Geometry: final body of the model. Coordinates: model frame, mm. A direction names the side the tool comes from. Round coordinates to 2 decimals unless told otherwise and drop trailing zeros. Loops run counter-clockwise (first coordinate to the right, second up) from the corner with the lowest first, then second, coordinate; pieces in that order, holes last. Notation, with made-up numbers: M 83.5,-32 L 126.5,-32 A31 cw 126.5,-7 Z; hole C 79,-4.75 d3. An arc over 180 degrees is marked long. Answer as a JSON object with one key per item and string values.
Autodesk Inventor part; units mm, degrees
ref_plane "YZ Plane" through (0, 0, 0) normal (1, 0, 0) x (0, 1, 0)
ref_plane "XZ Plane" through (0, 0, 0) normal (0, 1, 0) x (-1, 0, 0)
ref_plane "XY Plane" through (0, 0, 0) normal (0, 0, 1) x (1, 0, 0)
sketch "Sketch1" plane through (0, 0, 0) normal (0, 1, 0) x (-1, 0, 0)
  circle A0 centre (0, 0) radius 22.2885
  dimension "d0" = 44.577
extrude "Extrusion1" add sketch "Sketch1" along normal blind 12.7
chamfer "Chamfer1" distance 0.7384 angle 45 1 edges at (22.2885, 0, 0)
sketch "Sketch2" plane through (0, 12.7, 0) normal (0, 1, 0) x (1, 0, 0)
  circle A0 centre (0, 0) radius 16.002
  dimension "d6" = 32.004
extrude "Extrusion2" cut sketch "Sketch2" against normal blind 2.8702
sketch "Sketch3" plane through (0, 9.8298, 0) normal (0, 1, 0) x (1, 0, 0)
  circle A0 centre (0, 0) radius 8.3566
  circle A1 centre (0, 0) radius 7.0866
  dimension "d9" = 16.7132
  dimension "d10" = 1.27
extrude "Extrusion3" cut sketch "Sketch3" against normal blind 1.016
sketch "Sketch4" plane through (0, 9.8298, 0) normal (0, 1, 0) x (1, 0, 0)
  circle A0 centre (0, 0) radius 6.35
  dimension "d13" = 12.7
extrude "Extrusion4" cut sketch "Sketch4" against normal up to surface (9.8298 mm away)
chamfer "Chamfer2" distance 0.7384 angle 45 1 edges at (-6.35, 0, 0)
sketch "Sketch5" plane through (0, 9.8298, 0) normal (0, 1, 0) x (1, 0, 0)
  circle A0 centre (0, 0) radius 6.35
  circle A1 centre (0, 0) radius 5.715
  circle A2 centre (0, 0) radius 6.35
  dimension "d19" = 11.43
extrude "Extrusion5" add sketch "Sketch5" against normal blind 38.1
sketch "Sketch6" plane through (0, 12.7, 0) normal (0, 1, 0) x (1, 0, 0)
  line L0 (0, 0) -> (17.0477, 9.8425) construction
  line L1 (0, 0) -> (19.685, 0) construction
  dimension "d22" = 19.685
  dimension "d23" = 30
hole "Hole1" at (17.0477, 12.7, -9.8425) direction (0, -1, 0) diameter 3.175 end through all
chamfer "Chamfer3" distance 0.381 angle 45 1 edges at (17.0477, 12.7, -11.43)
pattern_circular "Circular Pattern1" count 12 over 360 about axis through (0, 0, 0) along (0, 1, 0) of "Hole1", "Chamfer3"
properties part number "universal connector" material "Stainless Steel AISI 304"
1) Pull-direction query (Z, two-part tool) for faces 1 (the flat face through (0, 0, -9)), 2 (the cylindrical face through (10.187, 6.073, 18.597)); classes: +Z half, -Z half, draft (parallel to the pull), parting line (faces both ways), or undercut.
Results:
{"face 1": "draft", "face 2": "undercut"}
2) Pin query (flat end, axial travel): P1, Ø4, axis at x = 0, z = 19.68, coming from the -Y side; P2, Ø12, axis at x = 7.5, y = -8.5, coming from the -Z side; P3, Ø1.9, axis at x = 9.84, z = 17.05, coming from the -Y side; P4, Ø8, axis at y = -23, z = 6, coming from the -X side. Return the tip coordinate at first contact, or that it passes through.
Results:
{"P1": "y = 0", "P2": "z = -6.17", "P3": "through", "P4": "x = -6.03"}
3) Section query B-B (y = -18). Return the cut outline in (x, z) (3 decimals), and give its area (3 significant figures).
Results:
{"outline": "C 0,0 d12.7; hole C 0,0 d11.43", "area": "24.1 mm2"}
4) Reachability of faces 3 (the cylindrical face through (0.48, 6.07, -21.2)), 4 (the cylindrical face through (-0.923, 9.329, -7.026)), 5 (the cylindrical face through (-1.38, -13.56, 6.2)) from +Z, -Z, +X, -X, +Y, -Y: full face, straight path, thin tool, end or side. Return the list, or none.
Results:
{"face 3": "+Y, -Y", "face 4": "+Y", "face 5": "-Y"}
5) Section query A-A (z = 0). Count the separate pieces of the cut face and the enclosed holes in it, and give its area (3 significant figures).
Results:
{"separate pieces": "4", "enclosed holes": "0", "area": "313 mm2"}
6) Ray query, line 1 (Z direction, x = -16, y = 6.5); line 2 (Y direction, x = -12.5, z = -9); line 3 (Y direction, x = 1, z = -6). Return the intervals inside material, ascending.
Results:
{"line 1": "-15.52 to -11.04, -8.65 to 8.65, 11.04 to 15.52", "line 2": "0 to 9.83", "line 3": "-28.27 to 9.83"}
